```python
from build123d import *

# Parameters (mm, degrees)
SKETCH_1_W          = 11.95
SKETCH_1_H          = 13.2
EXTRUDE_1_DEPTH     = 0.8
SKETCH_2_W          = 0.395
SKETCH_2_H          = 7.5
CUT_EXTRUDE_1_DEPTH = 0.8
CUT_EXTRUDE_2_DEPTH = 0.8
SKETCH_4_R          = 0.45
CUT_EXTRUDE_3_DEPTH = 0.8


with BuildPart() as part:
    # Эскиз1 → Бобышка-Вытянуть1 (new body)
    with BuildSketch(Plane.XY):
        Rectangle(SKETCH_1_W, SKETCH_1_H)
    extrude(amount=EXTRUDE_1_DEPTH)

    # Эскиз2 → Вырез-Вытянуть1 (cut)
    with BuildSketch(Plane.XY.offset(0.8)):
        with Locations((-5.7775, 2.85)):
            Rectangle(SKETCH_2_W, SKETCH_2_H)
        with Locations((5.7775, 2.85)):
            Rectangle(SKETCH_2_W, SKETCH_2_H)
    extrude(amount=-CUT_EXTRUDE_1_DEPTH, mode=Mode.SUBTRACT)

    # Эскиз3 → Вырез-Вытянуть2 (cut)
    with BuildSketch(Plane.XY.offset(0.8)):
        with BuildLine():
            Line((-5.2, 6.6), (-3.6, 6.6))
            ThreePointArc((-3.6, 6.6), (-4.4, 5.8), (-5.2, 6.6))
        make_face()
        with BuildLine():
            Line((-3, 6.6), (-1.4, 6.6))
            ThreePointArc((-1.4, 6.6), (-2.2, 5.8), (-3, 6.6))
        make_face()
        with BuildLine():
            Line((-0.8, 6.6), (0.8, 6.6))
            ThreePointArc((0.8, 6.6), (0, 5.8), (-0.8, 6.6))
        make_face()
        with BuildLine():
            Line((1.4, 6.6), (3, 6.6))
            ThreePointArc((3, 6.6), (2.2, 5.8), (1.4, 6.6))
        make_face()
        with BuildLine():
            Line((3.6, 6.6), (5.2, 6.6))
            ThreePointArc((5.2, 6.6), (4.4, 5.8), (3.6, 6.6))
        make_face()
    extrude(amount=-CUT_EXTRUDE_2_DEPTH, mode=Mode.SUBTRACT)

    # Эскиз4 → Вырез-Вытянуть3 (cut)
    with BuildSketch(Plane.XY.offset(0.8)):
        with Locations((-2.4, -5.4)):
            Circle(SKETCH_4_R)
        with Locations((0, -5.4)):
            Circle(SKETCH_4_R)
        with Locations((2.4, -5.4)):
            Circle(SKETCH_4_R)
        with Locations((-2.4, 0.025)):
            Circle(SKETCH_4_R)
        with Locations((0, 0.025)):
            Circle(SKETCH_4_R)
        with Locations((2.4, 0.025)):
            Circle(SKETCH_4_R)
        with Locations((-5.175, -5.4)):
            Circle(SKETCH_4_R)
        with Locations((5.175, -5.4)):
            Circle(SKETCH_4_R)
        with Locations((-4.4, 3.025)):
            Circle(SKETCH_4_R)
        with Locations((-2.2, 3.025)):
            Circle(SKETCH_4_R)
        with Locations((0, 3.025)):
            Circle(SKETCH_4_R)
        with Locations((2.2, 3.025)):
            Circle(SKETCH_4_R)
        with Locations((4.4, 3.025)):
            Circle(SKETCH_4_R)
    extrude(amount=-CUT_EXTRUDE_3_DEPTH, mode=Mode.SUBTRACT)


solid = part.part
```
Verification items for the finished model (mm, model axes). Round coordinates to 2 decimals unless told otherwise and drop trailing zeros. Write each loop counter-clockwise with the first axis right and the second up, starting at its lowest first coordinate (ties: lowest second). Pieces come first, ordered by that corner, then holes.
1. Draft check along X on faces 1 (the cylindrical face through (-2.19, -5.8, 0.41)), 2 (the flat face through (1, 0, 0.8)). Enter one of: +X half, -X half, draft (parallel to the pull), parting line (faces both ways), or undercut.
2. Section check C-C on x = -2.2. Enter the section's corners in (y, z) (3 decimals), plus the area to 3 significant figures.
3. Scan lines: L1, parallel to Y at x = 0, z = 0.6 (3 decimals); L2, parallel to Y at x = -4.4, z = 0.35 (3 decimals); L3, parallel to Y at x = 2.75, z = 0.75. Record each from-to range of solid material in increasing order.
4. Section check A-A on x = 4.4. Enter the section's corners in (y, z) (3 decimals).
5. Section check B-B on y = -5.4. Enter the section's corners in (x, z) (3 decimals).
6. Section check D-D on z = 0.55. State how many separate pieces and enclosed holes the cut face has, plus the area to 3 significant figures.
Answer:
1. face 1: undercut
1. face 2: draft
2. outline: (-6.6, 0) - (-5.803, 0) - (-5.803, 0.8) - (-6.6, 0.8) - close; (-4.997, 0) - (-0.378, 0) - (-0.378, 0.8) - (-4.997, 0.8) - close; (0.428, 0) - (2.575, 0) - (2.575, 0.8) - (0.428, 0.8) - close; (3.475, 0) - (5.8, 0) - (5.8, 0.8) - (3.475, 0.8) - close
2. area: 7.91 mm2
3. L1: y = -6.6 to -5.85, -4.95 to -0.425, 0.475 to 2.575, 3.475 to 5.8
3. L2: y = -6.6 to 2.575, 3.475 to 5.8
3. L3: y = -6.6 to -5.68, -5.12 to -0.26, 0.31 to 6.02
4. outline: (-6.6, 0) - (2.575, 0) - (2.575, 0.8) - (-6.6, 0.8) - close; (3.475, 0) - (5.8, 0) - (5.8, 0.8) - (3.475, 0.8) - close
5. outline: (-5.975, 0) - (-5.625, 0) - (-5.625, 0.8) - (-5.975, 0.8) - close; (-4.725, 0) - (-2.85, 0) - (-2.85, 0.8) - (-4.725, 0.8) - close; (-1.95, 0) - (-0.45, 0) - (-0.45, 0.8) - (-1.95, 0.8) - close; (0.45, 0) - (1.95, 0) - (1.95, 0.8) - (0.45, 0.8) - close; (2.85, 0) - (4.725, 0) - (4.725, 0.8) - (2.85, 0.8) - close; (5.625, 0) - (5.975, 0) - (5.975, 0.8) - (5.625, 0.8) - close
6. separate pieces: 1
6. enclosed holes: 13
6. area: 139 mm2
